For this review, take the finished solid that the model builds, in its own axes (mm). Face numbers are marked on the shaded views. A direction names the side the tool comes from. Coordinates: 2 decimals unless noted, no trailing zeros. Write each loop counter-clockwise with the first axis right and the second up, starting at its lowest first coordinate (ties: lowest second). Pieces come first, ordered by that corner, then holes.
Solid Edge part; units mm, degrees
sketch "Sketch1" plane through (0, 0, 0) normal (0, 0, 1) x (1, 0, 0)
  line L0 (6.5, -32) -> (6.5, -18)
  arc A0 (6.5, -18) -> (10, -7.5) centre (24, -18) cw
  arc A1 (-6.5, -18) -> (-10, -7.5) centre (-24, -18) ccw
  line L1 (-6.5, -18) -> (-6.5, -32)
  line L2 (-6.5, -32) -> (6.5, -32)
  arc A2 (-10, -7.5) -> (10, -7.5) centre (0, 0) cw
  circle A3 centre (0, 0) radius 9
extrude "Protrusion1" add sketch "Sketch1" along normal blind 4.5
sketch "Sketch2" plane through (0, -9.75, 4.5) normal (0, 0, 1) x (1, 0, 0)
  line L0 (5, -20.75) -> (5, -9.75)
  line L1 (5, -9.75) -> (-5, -9.75)
  line L2 (-5, -9.75) -> (-5, -20.75)
  line L3 (-5, -20.75) -> (5, -20.75)
  line L4 (6.5, -22.25) -> (6.5, -8.25)
  line L5 (6.5, -8.25) -> (-6.5, -8.25)
  line L6 (-6.5, -8.25) -> (-6.5, -22.25)
  line L7 (-6.5, -22.25) -> (6.5, -22.25)
extrude "ExtrudedProtrusion_2" add sketch "Sketch2" along normal blind 40
extrude "Cutout1" [suppressed]
sketch "Sketch3" plane through (0, -2.75, 4.5) normal (0, 0, 1) x (1, 0, 0)
  line L0 (-14.9811, 5.708) -> (-5.4512, 20.4845)
  line L1 (-5.4512, 20.4845) -> (11.5832, 18.4165)
  line L2 (11.5832, 18.4165) -> (13.7791, 5.708)
  line L3 (13.7791, 5.708) -> (8.5, 5.708)
  line L4 (-8.5, 5.708) -> (8.5, 5.708)
  line L5 (-8.5, 5.708) -> (-14.9811, 5.708)
extrude "Cutout2" cut sketch "Sketch3" against normal through all
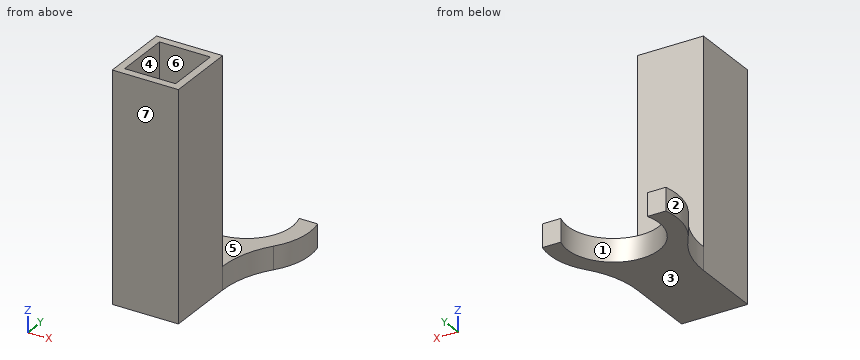
1) For L1, parallel to X at y = 0, z = 1.3; L2, parallel to Y at x = -1, z = 29.5; L3, parallel to X at y = -21.5, z = 19, list the stretches that pass through material, from the lowest coordinate up.
2) Consider section D-D (y = -28.5). Give the boundary of the cut face in (x, z), then the cut area to 4 significant figures.
3) Consider section A-A (y = 0). Give the boundary of the cut face in (x, z).
4) Consider section C-C (z = 23). Give the boundary of the cut face in (x, y), then the cut area to 3 significant figures.
5) Consider section B-B (x = 0). Give the boundary of the cut face in (y, z).
6) Clearance check with flat-ended pins moving along their axes: P1, Ø6, axis at x = -6.5, z = 20.5, coming from the +Y side; P2, Ø9, axis at y = -26, z = 20, coming from the +X side; P3, Ø12, axis at y = -25, z = 18, coming from the -X side. State where each tip first meets the part, or that it passes through.
7) Tool access review of the marked faces 5, 6 and 7: name each direction out of +Z, -Z, +X, -X, +Y, -Y from which nothing blocks a thin tool from reaching the whole face with its end or side.
8) The part is to be moulded in two halves that separate along X. For the marked faces 1, 2, 3 and 4, say which applies: pulls with the +X half, pulls with the -X half, needs draft (parallel to the pull), parting line crosses it, or undercut.
Results:
1. L1: x = -12.5 to -9, 9 to 12.5
1. L2: y = -32 to -30.5, -19.5 to -18
1. L3: x = -6.5 to -5, 5 to 6.5
2. outline: (-6.5, 0) - (6.5, 0) - (6.5, 44.5) - (5, 44.5) - (5, 4.5) - (-5, 4.5) - (-5, 44.5) - (-6.5, 44.5) - close
2. area: 178.5 mm2
3. outline: (-12.5, 0) - (-9, 0) - (-9, 4.5) - (-12.5, 4.5) - close; (9, 0) - (12.5, 0) - (12.5, 4.5) - (9, 4.5) - close
4. outline: (-6.5, -32) - (6.5, -32) - (6.5, -18) - (-6.5, -18) - close; hole (-5, -30.5) - (5, -30.5) - (5, -19.5) - (-5, -19.5) - close
4. area: 72.0 mm2
5. outline: (-32, 0) - (-9, 0) - (-9, 4.5) - (-18, 4.5) - (-18, 44.5) - (-19.5, 44.5) - (-19.5, 4.5) - (-30.5, 4.5) - (-30.5, 44.5) - (-32, 44.5) - close
6. P1: stops at y = -18
6. P2: stops at x = 6.5
6. P3: stops at x = -6.5
7. face 5: +Z, +X, -X, +Y
7. face 6: +Z
7. face 7: +Z, -Z, +X, -X, -Y
8. face 1: undercut
8. face 2: pulls with the -X half
8. face 3: needs draft
8. face 4: undercut
